Work out the finished part from the listing and answer in its coordinate system (mm). Coordinates: 2 decimals unless noted, no trailing zeros. Loops run counter-clockwise (first coordinate to the right, second up) from the corner with the lowest first, then second, coordinate; pieces in that order, holes last. Notation, with made-up numbers: (28.5, -10) -> (60.5, -10) arc R11 ccw to (60.5, 8) -> close; hole circle Ø2 at (31, -32.75). An arc over 180 degrees is marked (long way). Use a Markdown table: item, result. Add a question column.
```python
from build123d import *

# Parameters (mm, degrees)
CROQUIS1_W              = 320
CROQUIS1_H              = 158
CROQUIS1_R              = 18.764717073
SALIENTE_EXTRUIR1_DEPTH = 25.4


with BuildPart() as part:
    # Croquis1 → Saliente-Extruir1 (new body)
    with BuildSketch(Plane.XY):
        with Locations((0, 21)):
            Rectangle(CROQUIS1_W, CROQUIS1_H)
        Circle(CROQUIS1_R, mode=Mode.SUBTRACT)
        with Locations((110, 0)):
            Circle(CROQUIS1_R, mode=Mode.SUBTRACT)
        with Locations((-110, 0)):
            Circle(CROQUIS1_R, mode=Mode.SUBTRACT)
    extrude(amount=SALIENTE_EXTRUIR1_DEPTH)


solid = part.part
```
Item 1: Section D-D (x = -1.5) is taken. Determine the outline of the cut face in (y, z).
Item 2: Section B-B (y = 0) is taken. Determine the outline of the cut face in (x, z).
Item 3: Find the intervals of material crossed by probe 1 along Y at (x, z) = (-110, 18); probe 2 along X at (y, z) = (14, 15); probe 3 along X at (y, z) = (-15.5, 7), in increasing order.
Item 4: Section A-A (x = -110) is taken. Determine the outline of the cut face in (y, z).
Item 5: Given pin 1 (5 mm diameter, centred on x = -55.5, y = 31.5, fed in from -Z), flat-ended and moving along its own axis, determine where the tip first touches the part or whether it passes through.
Item 6: For a pull along X with two mould halves and no side action, classify faces 1 (the face through (-160, 20, 13)), 2 (the face through (-2, -58, 13)), 3 (the face through (127.898, 5.636, 12.522)), 4 (the face through (-92.102, 5.636, 12.522)) as +X half, -X half, draft (parallel to the pull), parting line (faces both ways), or undercut.
Item 7: Section C-C (z = 15.25) is taken. Determine the outline of the cut face in (x, y).
Output:
| question | item | result |
|---|---|---|
| 1 | outline | (-58, 0) -> (-18.7, 0) -> (-18.7, 25.4) -> (-58, 25.4) -> close; (18.7, 0) -> (100, 0) -> (100, 25.4) -> (18.7, 25.4) -> close |
| 2 | outline | (-160, 0) -> (-128.76, 0) -> (-128.76, 25.4) -> (-160, 25.4) -> close; (-91.24, 0) -> (-18.76, 0) -> (-18.76, 25.4) -> (-91.24, 25.4) -> close; (18.76, 0) -> (91.24, 0) -> (91.24, 25.4) -> (18.76, 25.4) -> close; (128.76, 0) -> (160, 0) -> (160, 25.4) -> (128.76, 25.4) -> close |
| 3 | probe 1 | y = -58 to -18.76, 18.76 to 100 |
| 3 | probe 2 | x = -160 to -122.49, -97.51 to -12.49, 12.49 to 97.51, 122.49 to 160 |
| 3 | probe 3 | x = -160 to -120.58, -99.42 to -10.58, 10.58 to 99.42, 120.58 to 160 |
| 4 | outline | (-58, 0) -> (-18.76, 0) -> (-18.76, 25.4) -> (-58, 25.4) -> close; (18.76, 0) -> (100, 0) -> (100, 25.4) -> (18.76, 25.4) -> close |
| 5 | pin 1 | stops at z = 0 |
| 6 | face 1 | -X half |
| 6 | face 2 | draft |
| 6 | face 3 | undercut |
| 6 | face 4 | undercut |
| 7 | outline | (-160, -58) -> (160, -58) -> (160, 100) -> (-160, 100) -> close; hole circle Ø37.53 at (-110, 0); hole circle Ø37.53 at (0, 0); hole circle Ø37.53 at (110, 0) |
